```python
from build123d import *

# Parameters (mm, degrees)
SKETCH_1_R           = 5.95
EXTRUDE_1_DEPTH      = 4.5
SKETCH_4_R           = 8.45
EXTRUDE_4_DEPTH      = 17.75
EXTRUDE_6_DEPTH      = 5.75
EXTRUDE_6_DEPTH_BACK = 5.75
SKETCH_12_R          = 9.5
EXTRUDE_10_DEPTH     = 1
SKETCH_7_R           = 2.3
CUT_EXTRUDE_1_DEPTH  = 57.22806055
SKETCH_8_R           = 6.5
CUT_EXTRUDE_2_DEPTH  = 6
SKETCH_9_R           = 9.5
EXTRUDE_7_DEPTH      = 36
SKETCH_10_R          = 8.45
EXTRUDE_8_DEPTH      = 40
EXTRUDE_START        = 1
SKETCH_13_R          = 9.5
SKETCH_13_R_2        = 2.3
EXTRUDE_11_DEPTH     = 1
SKETCH_14_R          = 3.25
CUT_EXTRUDE_3_DEPTH  = 8
CUT_EXTRUDE_START    = -18
CUT_EXTRUDE_4_DEPTH  = 18
CUT_EXTRUDE_START_2  = 11
SKETCH_16_R          = 14.956390748
SKETCH_16_R_2        = 7.5
CUT_EXTRUDE_5_DEPTH  = 22
FILLET_2_R           = 5
SKETCH_17_R          = 7.5
EXTRUDE_12_DEPTH     = 11.5


with BuildPart() as part:
    # Эскиз1 → Бобышка-Вытянуть1 (new body)
    with BuildSketch(Plane(origin=(0, 0, 0), x_dir=(1, 0, 0), z_dir=(0, 1, 0))):
        with Locations(Location((0, 0, 0), (0, 0, 270))):
            Circle(SKETCH_1_R)
    extrude(amount=EXTRUDE_1_DEPTH)

    # Эскиз4 → Бобышка-Вытянуть4 (add)
    with BuildSketch(Plane(origin=(0, 4.5, 0), x_dir=(1, 0, 0), z_dir=(0, 1, 0))):
        with Locations(Location((0, 0, 0), (0, 0, 270))):
            Circle(SKETCH_4_R)
    extrude(amount=EXTRUDE_4_DEPTH)

    # Эскиз6 → Бобышка-Вытянуть6 (add, two sides: drawn at the far end of the back side and taken through both)
    with BuildSketch(Plane(origin=(0, 22.25, 0), x_dir=(1, 0, 0), z_dir=(0, 1, 0)).offset(-EXTRUDE_6_DEPTH_BACK)):
        with BuildLine():
            Line((0, -9.5), (-0.833655922, -9.5))
            ThreePointArc((-0.833655922, -9.5), (-3.331132848, -9.18310947), (-5.670324417, -8.252521801))
            ThreePointArc((-5.670324417, -8.252521801), (-13.556905273, -2.05094269), (-19.066851837, 6.333461279))
            Line((-19.066851837, 6.333461279), (-28.114764095, 31.1923959))
            Line((-28.114764095, 31.1923959), (-10.2606043, 37.690778624))
            Line((-10.2606043, 37.690778624), (-2.394850826, 16.079798567))
            ThreePointArc((-2.394850826, 16.079798567), (1.266311019, 11.308479557), (7.002075382, 9.5))
            Line((7.002075382, 9.5), (30, 9.5))
            Line((30, 9.5), (30, -9.5))
            Line((30, -9.5), (0, -9.5))
        make_face()
    extrude(amount=EXTRUDE_6_DEPTH + EXTRUDE_6_DEPTH_BACK)

    # Эскиз12 → Бобышка-Вытянуть10 (add)
    with BuildSketch(Plane(origin=(0, 28, 0), x_dir=(1, 0, 0), z_dir=(0, 1, 0))):
        with Locations(Location((-15.938492836, 25.514507365, 0), (0, 0, 110))):
            Circle(SKETCH_12_R)
    extrude(amount=EXTRUDE_10_DEPTH)

    # Эскиз7 → Вырез-Вытянуть1 (cut, through all)
    with BuildSketch(Plane.XZ):
        with Locations(Location((0, 0, 0), (0, 0, 270))):
            Circle(SKETCH_7_R)
    extrude(amount=-CUT_EXTRUDE_1_DEPTH, mode=Mode.SUBTRACT)

    # Эскиз8 → Вырез-Вытянуть2 (cut)
    with BuildSketch(Plane(origin=(0, 28, 0), x_dir=(1, 0, 0), z_dir=(0, 1, 0))):
        with Locations(Location((0, 0, 0), (0, 0, 270))):
            Circle(SKETCH_8_R)
    extrude(amount=-CUT_EXTRUDE_2_DEPTH, mode=Mode.SUBTRACT)

    # Эскиз9 → Бобышка-Вытянуть7 (add)
    with BuildSketch(Plane.XZ.offset(-28)):
        with Locations(Location((20.5, 0, 0), (0, 0, 90))):
            Circle(SKETCH_9_R)
    extrude(amount=-EXTRUDE_7_DEPTH)

    # Эскиз10 → Бобышка-Вытянуть8 (add)
    with BuildSketch(Plane(origin=(0, 29, 0), x_dir=(1, 0, 0), z_dir=(0, 1, 0))):
        with Locations(Location((-15.938492836, 25.514507365, 0), (0, 0, 270))):
            Circle(SKETCH_10_R)
    extrude(amount=EXTRUDE_8_DEPTH)

    # Эскиз13 → Бобышка-Вытянуть11 (add)
    with BuildSketch(Plane.XZ.offset(-16.5).offset(EXTRUDE_START)):
        with Locations(Location((0, 0, 0), (0, 0, 90))):
            Circle(SKETCH_13_R)
        with Locations(Location((0, 0, 0), (0, 0, 270))):
            Circle(SKETCH_13_R_2, mode=Mode.SUBTRACT)
    extrude(amount=-EXTRUDE_11_DEPTH)

    # Эскиз14 → Вырез-Вытянуть3 (cut)
    with BuildSketch(Plane(origin=(0, 69, 0), x_dir=(1, 0, 0), z_dir=(0, 1, 0))):
        with Locations(Location((-15.938492836, 25.514507365, 0), (0, 0, 270))):
            Circle(SKETCH_14_R)
    extrude(amount=-CUT_EXTRUDE_3_DEPTH, mode=Mode.SUBTRACT)

    # Эскиз15 → Вырез-Вытянуть4 (cut)
    with BuildSketch(Plane(origin=(0, 28, 0), x_dir=(1, 0, 0), z_dir=(0, 1, 0)).offset(CUT_EXTRUDE_START)):
        with BuildLine():
            Line((-24.865572733, 22.265316003), (-35.336248809, 21.155444764))
            Line((-35.336248809, 21.155444764), (-35.336248809, 37.040132254))
            Line((-35.336248809, 37.040132254), (1.913807819, 42.427920993))
            Line((1.913807819, 42.427920993), (-7.011412938, 28.763698726))
            ThreePointArc((-7.011412938, 28.763698726), (-19.187684197, 34.441587262), (-24.865572733, 22.265316003))
        make_face()
        with BuildLine():
            Line((20.5, 9.5), (21.51421168, 16.603692208))
            Line((21.51421168, 16.603692208), (46.391879719, 13.051846104))
            Line((46.391879719, 13.051846104), (43.436938274, -14.794111134))
            Line((43.436938274, -14.794111134), (20.5, -14.236753678))
            Line((20.5, -14.236753678), (20.5, -9.5))
            ThreePointArc((20.5, -9.5), (30, 0), (20.5, 9.5))
        make_face()
    extrude(amount=CUT_EXTRUDE_4_DEPTH, mode=Mode.SUBTRACT)

    # Эскиз16 → Вырез-Вытянуть5 (cut)
    with BuildSketch(Plane(origin=(0, 28, 0), x_dir=(1, 0, 0), z_dir=(0, 1, 0)).offset(CUT_EXTRUDE_START_2)):
        with Locations((20.5, 0)):
            Circle(SKETCH_16_R)
        with Locations(Location((20.5, 0, 0), (0, 0, 270))):
            Circle(SKETCH_16_R_2, mode=Mode.SUBTRACT)
    extrude(amount=CUT_EXTRUDE_5_DEPTH, mode=Mode.SUBTRACT)

    # Скругление2
    # the kernel refuses this fillet: 5 mm, written as the material it adds along each edge
    with BuildSketch(Plane(origin=(20.5, 39, 0), x_dir=(0, 0, 1), z_dir=(-1, 0, 0))) as fillet_2_piece_1:
        with BuildLine():
            CenterArc((12.5, 4), FILLET_2_R, 180, 53.130102354)
            Line((7.5, 4), (7.4, 4))
            Line((7.4, 4), (7.4, 0))
            Line((7.4, 0), (7.5, -0.1))
            ThreePointArc((7.5, -0.1), (8.5, -0.1), (9.44, -0.08))
            Line((9.44, -0.08), (9.5, 0))
        make_face()
    revolve(axis=Axis((20.5, 39, 0), (0, 1, 0)))
    with BuildSketch(Plane(origin=(20.5, 61, 0), x_dir=(0, 0, 1), z_dir=(-1, 0, 0))) as fillet_2_piece_2:
        with BuildLine():
            CenterArc((12.5, -4), FILLET_2_R, 126.869897646, 53.130102354)
            Line((9.5, 0), (9.44, 0.08))
            ThreePointArc((9.44, 0.08), (8.5, 0.1), (7.5, 0.1))
            Line((7.5, 0.1), (7.4, 0))
            Line((7.4, 0), (7.4, -4))
            Line((7.4, -4), (7.5, -4))
        make_face()
    revolve(axis=Axis((20.5, 61, 0), (0, 1, 0)))

    # Эскиз17 → Бобышка-Вытянуть12 (add)
    with BuildSketch(Plane(origin=(0, 28, 0), x_dir=(1, 0, 0), z_dir=(0, 1, 0))):
        with BuildLine():
            Line((-9.278482036, -11.69085434), (-12.972576627, -8.775389277))
            ThreePointArc((-12.972576627, -8.775389277), (-20.997261978, 0.921608959), (-24.337711873, 13.057042378))
            Line((-24.337711873, 13.057042378), (-24.865572733, 22.265316003))
            Line((-24.865572733, 22.265316003), (-5.413533881, 23.476451416))
            Line((-5.413533881, 23.476451416), (9.371872764, 11.807465836))
            ThreePointArc((9.371872764, 11.807465836), (8.040562687, -6.286337643), (-9.278482036, -11.69085434))
        make_face()
        Circle(SKETCH_17_R, mode=Mode.SUBTRACT)
    extrude(amount=-EXTRUDE_12_DEPTH)


solid = part.part
```
Source: CAD feature listing. Evaluate the final solid. Frame: model axes, mm. A direction names the side the tool comes from. Give positions to 0.01 mm unless a question says otherwise; leave off trailing zeros. Order: outer loops, then holes, each group sorted by start corner. A loop starts at its lowest first (then second) coordinate and runs counter-clockwise, first axis right, second up.
(1) Access query for faces 4 (the face through (0, 22, 3)), 5 (the face through (-24.6, 22.3, -17.6)), 6 (the face through (5.78, 15.99, -7.54)). Directions: +Z, -Z, +X, -X, +Y, -Y. A direction counts if a zero-diameter tool reaches every point of the face in a straight line with its end or side. Return the directions, or none.
(2) Section query C-C (y = 8.5). Return the cut outline in (x, z), plus the area to 3 significant figures.
(3) Contact query for flat-ended pins moving along their axis: P1, Ø12.5, axis at x = -7.5, z = 1.5, coming from the +Y side; P2, Ø1, axis at y = 35.5, z = -28, coming from the +X side; P3, Ø10, axis at y = 60.5, z = -7, coming from the -X side. Output: stop coordinate, or through.
(4) Section query D-D (x = -18). Return the cut outline in (y, z), plus the area to 3 significant figures.
(5) Pull-direction query (Y, two-part tool) for faces 1 (the face through (20, 64, 0)), 2 (the face through (27.936, 49.902, -0.976)), 3 (the face through (2.54, 9.92, 8.06)); classes: +Y half, -Y half, draft (parallel to the pull), parting line (faces both ways), or undercut.
(6) Section query B-B (x = 0). Return the cut outline in (y, z).
(7) Material intervals for line 1 along Y through (x, z) = (-19, -13.5); line 2 along Y through (x, z) = (25, 8); line 3 along Z through (x, y) = (20, 39), sorted ascending.
Outcome:
1. face 4: +Y
1. face 5: +Z, -X, +Y, -Y
1. face 6: -Y
2. outline: circle Ø16.9 at (0, 0); hole circle Ø4.6 at (0, 0)
2. area: 208 mm2
3. P1: stops at y = 28
3. P2: stops at x = -7.73
3. P3: stops at x = 11.22
4. outline: (16.5, -34.79) - (29, -34.79) - (29, -33.71) - (69, -33.71) - (69, -28.03) - (61, -28.03) - (61, -23) - (69, -23) - (69, -17.32) - (29, -17.32) - (29, -16.24) - (28, -16.24) - (28, 3.73) - (16.5, 3.73) - close
4. area: 1,080 mm2
5. face 1: +Y half
5. face 2: undercut
5. face 3: draft
6. outline: (0, -5.95) - (4.5, -5.95) - (4.5, -8.45) - (15.5, -8.45) - (15.5, -9.5) - (16.5, -9.5) - (16.5, -19.2) - (28, -19.2) - (28, -6.5) - (22, -6.5) - (22, -2.3) - (0, -2.3) - close; (0, 2.3) - (22, 2.3) - (22, 6.5) - (28, 6.5) - (28, 11.72) - (16.5, 11.72) - (16.5, 9.5) - (15.5, 9.5) - (15.5, 8.45) - (4.5, 8.45) - (4.5, 5.95) - (0, 5.95) - close
7. line 1: y = 16.5 to 28
7. line 2: y = 16.5 to 39.26, 60.74 to 64
7. line 3: z = -9.49 to 9.49
